```python
from build123d import *

# Parameters (mm, degrees)
F0_R     = 19
F1_DEPTH = 132
F2_R     = 5
F3_R     = 7.5
F4_DEPTH = 5
F5_R     = 2


with BuildPart() as f1:
    # F0 (on Front) → F1 (new body)
    with BuildSketch(Plane.XZ):
        Circle(F0_R)
    extrude(amount=F1_DEPTH)

    # F2
    f2_edges = [f1.edges().sort_by_distance(p)[0] for p in [
        (-19, -132, 0),
        (-19, 0, 0),
    ]]
    fillet(f2_edges, radius=F2_R)

    # F3 (on face) → F4 (join)
    with BuildSketch(Plane(origin=(0, 0, 0), x_dir=(-1, 0, 0), z_dir=(0, 1, 0))):
        Circle(F3_R)
    extrude(amount=F4_DEPTH)

    # F5
    f5_edges = [f1.edges().sort_by_distance(p)[0] for p in [
        (7.5, 5, 0),
    ]]
    fillet(f5_edges, radius=F5_R)


solid = f1.part
```
Work out the finished part from the listing and answer in its coordinate system (mm). A direction names the side the tool comes from. Round coordinates to 2 decimals unless told otherwise and drop trailing zeros. Write each loop counter-clockwise with the first axis right and the second up, starting at its lowest first coordinate (ties: lowest second). Pieces come first, ordered by that corner, then holes.
1) A cutting plane is placed at D-D on y = -3.5. Determine the outline of the cut face in (x, z), and give its area (3 significant figures).
2) A cutting plane is placed at A-A on z = 0. Determine the outline of the cut face in (x, y), and give its area (3 significant figures).
3) Flat-ended cylindrical pins translate along their axes: P1, Ø4, axis at x = -2.5, y = -39, coming from the -Z side; P2, Ø2, axis at x = -6.5, y = -16.5, coming from the -Z side; P3, Ø2, axis at x = 5, y = -74, coming from the +Z side; P4, Ø10, axis at y = -72, z = 4, coming from the -X side. Find the tip coordinate at first contact, or state that the pin passes through.
4) A cutting plane is placed at C-C on y = -31.5. Determine the outline of the cut face in (x, z).
5) Which of the six approach directions +Z, -Z, +X, -X, +Y, -Y give full straight-line access (tool end or side, diameter ignored) to faces 1 (the face through (6, 0, -6)), 2 (the face through (8.767, -65.146, -16.856))?
6) Consider probe 1 along Z at (x, y) = (1, -24.5); probe 2 along Y at (x, z) = (8, -8); probe 3 along X at (y, z) = (-119.5, -6). Determine where each line is inside the solid, lowest interval first.
7) A cutting plane is placed at B-B on x = 0. Determine the outline of the cut face in (y, z), and give its area (3 significant figures).
Entries:
1. outline: circle Ø37.54 at (0, 0)
1. area: 1,110 mm2
2. outline: (-19, -127) arc R5 ccw to (-14, -132) - (14, -132) arc R5 ccw to (19, -127) - (19, -5) arc R5 ccw to (14, 0) - (7.5, 0) - (7.5, 3) arc R2 ccw to (5.5, 5) - (-5.5, 5) arc R2 ccw to (-7.5, 3) - (-7.5, 0) - (-14, 0) arc R5 ccw to (-19, -5) - close
2. area: 5,070 mm2
3. P1: stops at z = -18.99
3. P2: stops at z = -18.19
3. P3: stops at z = 18.57
3. P4: stops at x = -19
4. outline: circle Ø38 at (0, 0)
5. face 1: +Y
5. face 2: +Y, -Y
6. probe 1: z = -18.97 to 18.97
6. probe 2: y = -132 to 0
6. probe 3: x = -18.03 to 18.03
7. outline: (-132, -14) arc R5 ccw to (-127, -19) - (-5, -19) arc R5 ccw to (0, -14) - (0, -7.5) - (3, -7.5) arc R2 ccw to (5, -5.5) - (5, 5.5) arc R2 ccw to (3, 7.5) - (0, 7.5) - (0, 14) arc R5 ccw to (-5, 19) - (-127, 19) arc R5 ccw to (-132, 14) - close
7. area: 5,070 mm2
